Read the model definition and answer for the solid it produces. Units are mm, in the model's axes. Give positions to 0.01 mm unless a question says otherwise; leave off trailing zeros. Order: outer loops, then holes, each group sorted by start corner. A loop starts at its lowest first (then second) coordinate and runs counter-clockwise, first axis right, second up. Notation, with made-up numbers: M 79,78 L 138,78 A21 cw 138,96 Z; hole C -14,9.25 d1. An arc over 180 degrees is marked long. One line per item, written item: value. Start each with the question number.
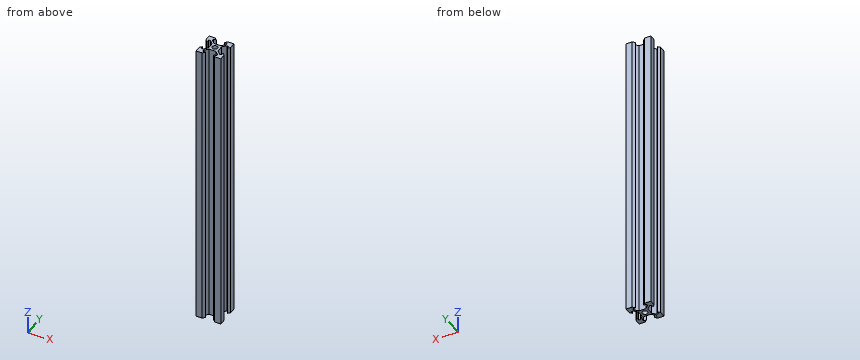
from build123d import *

# Parameters (mm, degrees)
CROQUIS1_R              = 2.15
SALIENTE_EXTRUIR2_DEPTH = 238


with BuildPart() as part:
    # Croquis1 → Saliente-Extruir2 (new body)
    with BuildSketch(Plane.XY):
        Polygon((4.4, 0), (0, 0), (0, -0.56736664), (0, -4.4), (0, -4.95), (1.8, -6.75), (1.8, -4.4), (3.410050506, -4.4), (6.175, -7.164949494), (6.175, -12.835050506), (3.410050506, -15.6), (1.8, -15.6), (1.8, -13.25), (0, -15.05), (0, -15.6), (0, -20), (4.4, -20), (4.95, -20), (6.75, -18.2), (4.4, -18.2), (4.4, -16.589949494), (7.164949494, -13.825), (12.835050506, -13.825), (15.6, -16.589949494), (15.6, -18.2), (13.25, -18.2), (15.05, -20), (15.6, -20), (18.2, -20), (20, -20), (20, -15.6), (20, -15.05), (18.2, -13.25), (18.2, -15.6), (16.589949494, -15.6), (13.825, -12.835050506), (13.825, -7.164949494), (16.589949494, -4.4), (18.2, -4.4), (18.2, -6.75), (20, -4.95), (20, -4.4), (20, 0), (15.6, 0), (15.05, 0), (13.25, -1.8), (15.6, -1.8), (15.6, -3.410050506), (12.835050506, -6.175), (7.164949494, -6.175), (4.4, -3.410050506), (4.4, -1.8), (6.75, -1.8), (4.95, 0), align=None)
        with Locations((10, -10)):
            Circle(CROQUIS1_R, mode=Mode.SUBTRACT)
    extrude(amount=SALIENTE_EXTRUIR2_DEPTH)


solid = part.part
Q1. Each of these flat-tipped pins is pushed along its axis until it touches: pin 1 (1.2 mm diameter, centred on x = 6, z = 165, fed in from +Y); pin 2 (12 mm diameter, centred on x = 15, y = -12.5, fed in from +Z); pin 3 (0.7 mm diameter, centred on x = 6, z = 106, fed in from -Y); pin 4 (6 mm diameter, centred on x = 9.5, z = 104, fed in from +Y). Where does it stop, or does it pass through?
Q2. Find section A-A, the plane x = 10. Give the vertices of the cut face in (y, z) (3 decimals).
Q3. Find section B-B, the plane y = -10. Give the vertices of the cut face in (x, z) (3 decimals), then the cut area to 3 significant figures.
Q4. Consider probe 1 along X at (y, z) = (-17.5, 29); probe 2 along Y at (x, z) = (10, 183) (3 decimals); probe 3 along Y at (x, z) = (14, 208). Determine where each line is inside the solid, lowest interval first.
Evaluation:
1. pin 1: y = -0.45
1. pin 2: z = 238
1. pin 3: y = -19.3
1. pin 4: y = -1.55
2. outline: M -13.825,0 L -12.15,0 L -12.15,238 L -13.825,238 Z; M -7.85,0 L -6.175,0 L -6.175,238 L -7.85,238 Z
3. outline: M 6.175,0 L 7.85,0 L 7.85,238 L 6.175,238 Z; M 12.15,0 L 13.825,0 L 13.825,238 L 12.15,238 Z
3. area: 797 mm2
4. probe 1: 0 to 4.4, 15.6 to 20
4. probe 2: -13.825 to -12.15, -7.85 to -6.175
4. probe 3: -18.95 to -18.2, -14.99 to -13.01, -6.99 to -5.01, -1.8 to -1.05
